The figure shows three views and two pictorial views of one solid part (mm, origin at its lowest corner). Answer the questions. A direction names the side the tool comes from. Give positions to 0.01 mm unless a question says otherwise; leave off trailing zeros. Order: outer loops, then holes, each group sorted by start corner. A loop starts at its lowest first (then second) coordinate and runs counter-clockwise, first axis right, second up. Notation, with made-up numbers: M 8.25,-5 L 66.25,-5 A20 ccw 66.25,24 Z; hole C 55,55 d1. An arc over 180 degrees is marked long. One line per item, written item: value.
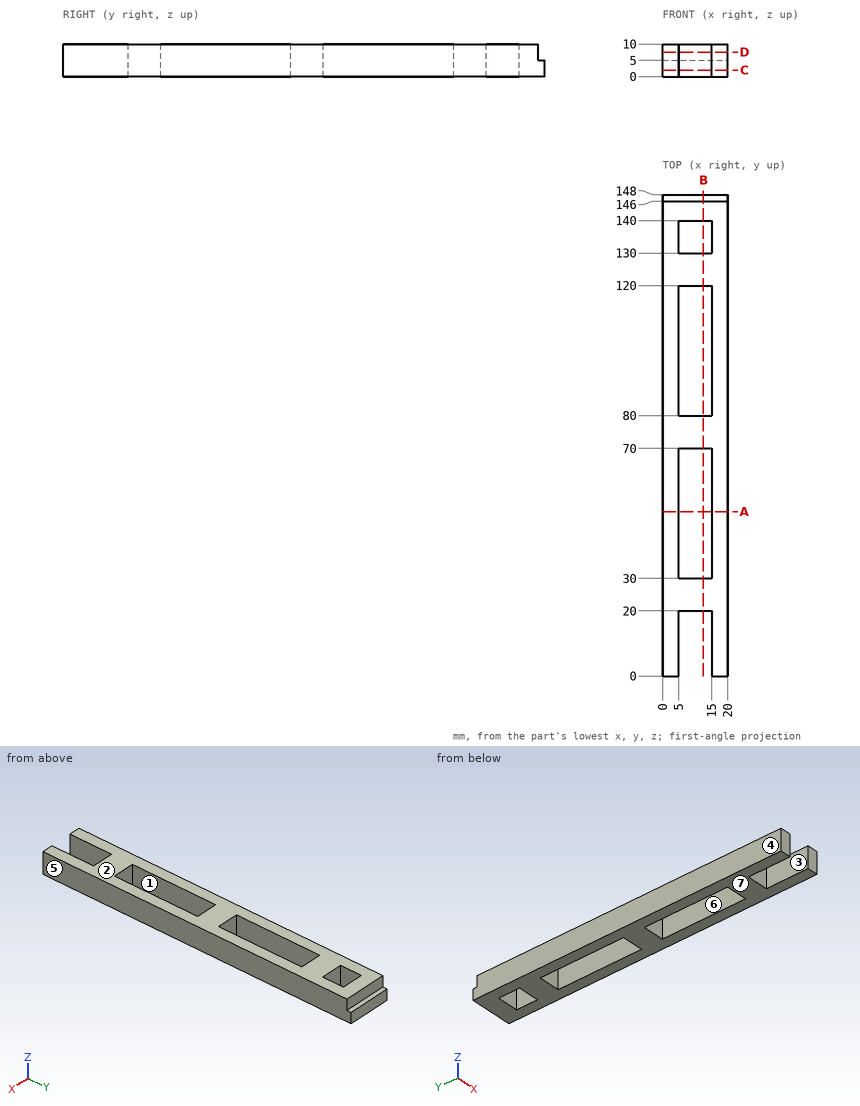
1) Find section A-A, the plane y = 50.5. Write down the section's boundary in (x, z), plus the area to 3 significant figures.
Reported:
outline: M 0,0 L 5,0 L 5,10 L 0,10 Z; M 15,0 L 20,0 L 20,10 L 15,10 Z
area: 100 mm^2
2) Determine the mould class of the marked faces 4, 5, 6 and 7 for opening direction X: +X half, -X half, draft (parallel to the pull), parting line (faces both ways), or undercut.
Reported:
face 4: -X half
face 5: +X half
face 6: undercut
face 7: draft
3) Find section D-D, the plane z = 7.5. Write down the section's boundary in (x, y).
Reported:
outline: M 0,0 L 5,0 L 5,20 L 15,20 L 15,0 L 20,0 L 20,146 L 0,146 Z; hole M 5,30 L 15,30 L 15,70 L 5,70 Z; hole M 5,80 L 15,80 L 15,120 L 5,120 Z; hole M 5,130 L 15,130 L 15,140 L 5,140 Z
4) Which of the six approach directions +Z, -Z, +X, -X, +Y, -Y give full straight-line access (tool end or side, diameter ignored) to the marked faces 1, 2 and 3?
Reported:
face 1: +Z, -Z
face 2: +Z, +X, -X, +Y, -Y
face 3: +Z, -Z, -Y
5) Each of these flat-tipped pins is pushed along its axis until it touches: pin 1 Ø5 at (y, z) = (9.5, 4.5) entering from -X; pin 2 Ø2.5 at (x, z) = (14.5, 6.5) entering from +Y; pin 3 Ø0.6 at (x, y) = (7.5, 147) entering from +Z; pin 4 Ø3 at (x, z) = (11.5, 5.5) entering from -Y. Where does it stop, or does it pass through?
Reported:
pin 1: stops at x = 0
pin 2: stops at y = 146
pin 3: stops at z = 5
pin 4: stops at y = 20
6) Find section C-C, the plane z = 2. Write down the section's boundary in (x, y), plus the area to 3 significant figures.
Reported:
outline: M 0,0 L 5,0 L 5,20 L 15,20 L 15,0 L 20,0 L 20,148 L 0,148 Z; hole M 5,30 L 15,30 L 15,70 L 5,70 Z; hole M 5,80 L 15,80 L 15,120 L 5,120 Z; hole M 5,130 L 15,130 L 15,140 L 5,140 Z
area: 1,860 mm^2
7) Consider probe 1 along Y at (x, z) = (5.5, 6.25); probe 2 along Y at (x, z) = (9.25, 2.25); probe 3 along X at (y, z) = (18, 8.5). Determine where each line is inside the solid, lowest interval first.
Reported:
probe 1: y = 20 to 30, 70 to 80, 120 to 130, 140 to 146
probe 2: y = 20 to 30, 70 to 80, 120 to 130, 140 to 148
probe 3: x = 0 to 5, 15 to 20
8) Find section B-B, the plane x = 12.5. Write down the section's boundary in (y, z), plus the area to 3 significant figures.
Reported:
outline: M 20,0 L 30,0 L 30,10 L 20,10 Z; M 70,0 L 80,0 L 80,10 L 70,10 Z; M 120,0 L 130,0 L 130,10 L 120,10 Z; M 140,0 L 148,0 L 148,5 L 146,5 L 146,10 L 140,10 Z
area: 370 mm^2
